from build123d import *

# Parameters (mm, degrees)
SKIZZE1_W                          = 20
SKIZZE1_H                          = 20
AUFSATZ_LINEAR_AUSTRAGEN1_DEPTH    = 15
SKIZZE2_R                          = 2.5
SCHNITT_LINEAR_AUSTRAGEN1_DEPTH    = 7
SKIZZE4_R                          = 4
SCHNITT_LINEAR_AUSTRAGEN7_DEPTH    = 33.015621187
M3X0_5_GEWINDEBOHRUNG1_D           = 2.5
M3X0_5_GEWINDEBOHRUNG1_CSINK_D     = 3.05
M3X0_5_GEWINDEBOHRUNG1_CSINK_ANGLE = 90


with BuildPart() as part:
    # Skizze1 → Aufsatz-Linear austragen1 (new body)
    with BuildSketch(Plane(origin=(0, 0, 0), x_dir=(1, 0, 0), z_dir=(0, 1, 0))):
        with Locations((10, 10)):
            Rectangle(SKIZZE1_W, SKIZZE1_H)
    extrude(amount=AUFSATZ_LINEAR_AUSTRAGEN1_DEPTH)

    # Skizze2 → Schnitt-Linear austragen1 (cut)
    with BuildSketch(Plane.XY):
        with Locations((10, 7.5)):
            Circle(SKIZZE2_R)
    extrude(amount=-SCHNITT_LINEAR_AUSTRAGEN1_DEPTH, mode=Mode.SUBTRACT)

    # Skizze4 → Schnitt-Linear austragen7 (cut, through all)
    with BuildSketch(Plane(origin=(20, 0, 0), x_dir=(0, 0, -1), z_dir=(1, 0, 0))):
        with Locations((13, 7.5)):
            Circle(SKIZZE4_R)
    extrude(amount=-SCHNITT_LINEAR_AUSTRAGEN7_DEPTH, mode=Mode.SUBTRACT)

    # M3x0.5 Gewindebohrung1 (through all)
    with Locations(Plane(origin=(12, 15, 0), x_dir=(0, 0, 1), z_dir=(0, 1, 0))):
        with Locations((-3.5, -2), (-13, -2)):
            CounterSinkHole(M3X0_5_GEWINDEBOHRUNG1_D / 2, M3X0_5_GEWINDEBOHRUNG1_CSINK_D / 2, counter_sink_angle=M3X0_5_GEWINDEBOHRUNG1_CSINK_ANGLE)


solid = part.part
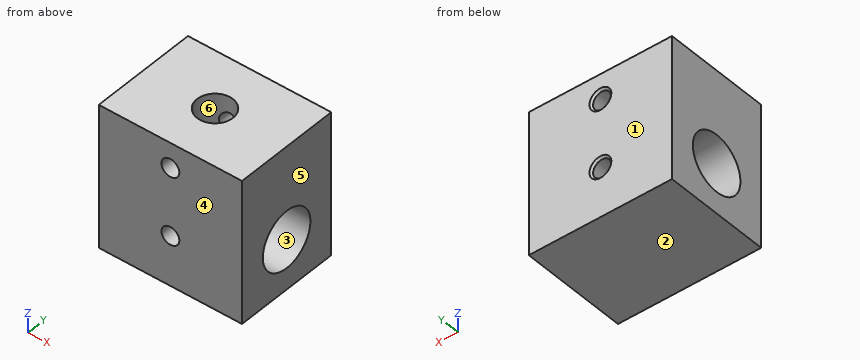
Part model, mm, in its own coordinate system. Face numbers are marked on the shaded views. A direction names the side the tool comes from. Give positions to 0.01 mm unless a question says otherwise; leave off trailing zeros. Loops run counter-clockwise (first coordinate to the right, second up) from the corner with the lowest first, then second, coordinate; pieces in that order, holes last.
(1) Band-saw the part on B-B (x = 10). Write the cut outline in (y, z) (3 decimals).
Return value:
outline: (0, -20) - (15, -20) - (15, -14.525) - (14.725, -14.25) - (11.3, -14.25) arc R4 cw to (3.7, -14.25) - (0, -14.25) - close; (0, -11.75) - (3.7, -11.75) arc R4 cw to (11.3, -11.75) - (14.725, -11.75) - (15, -11.475) - (15, -5.025) - (14.725, -4.75) - (10, -4.75) - (10, -7) - (5, -7) - (5, -4.75) - (0, -4.75) - close; (0, -2.25) - (5, -2.25) - (5, 0) - (0, 0) - close; (10, -2.25) - (14.725, -2.25) - (15, -1.975) - (15, 0) - (10, 0) - close
(2) Band-saw the part on A-A (y = 7.5). Write the cut outline in (x, z).
Return value:
outline: (0, -20) - (20, -20) - (20, -17) - (0, -17) - close; (0, -9) - (20, -9) - (20, 0) - (12.5, 0) - (12.5, -7) - (7.5, -7) - (7.5, 0) - (0, 0) - close
(3) Pull direction Y, two halves, no side cores. Call the marked faces 1, 2, 3 and 4: pulls with the +Y half, pulls with the -Y half, needs draft (parallel to the pull), parting line crosses it, or undercut.
Return value:
face 1: pulls with the +Y half
face 2: needs draft
face 3: undercut
face 4: pulls with the -Y half
(4) Drill centre lines: line 1 along Y through (x, z) = (7, -13); line 2 along X through (y, z) = (12.05, -13); line 3 along Z through (x, y) = (13.75, 6.25). Where is each one in solid material? Low to high.
Return value:
line 1: y = 0 to 3.5, 11.5 to 15
line 2: x = 0 to 8.75, 11.25 to 20
line 3: z = -20 to -16.8, -9.2 to 0
(5) 3-axis set-ups, long thin cutter, end or side, ignore diameter. For the marked faces 5 and 6: which of +Z, -Z, +X, -X, +Y, -Y reach the whole face in a straight line?
Return value:
face 5: +Z, -Z, +X, +Y, -Y
face 6: +Z
(6) Band-saw the part on D-D (x = 6.25). Write the cut outline in (y, z).
Return value:
outline: (0, -20) - (15, -20) - (15, 0) - (0, 0) - close; hole circle Ø8 at (7.5, -13)
(7) Band-saw the part on C-C (z = -3.5). Write the cut outline in (x, y) (3 decimals), and give its area (3 significant figures).
Return value:
outline: (0, 0) - (8.75, 0) - (8.75, 5.335) arc R2.5 cw to (8.75, 9.665) - (8.75, 14.725) - (8.475, 15) - (0, 15) - close; (11.25, 0) - (20, 0) - (20, 15) - (11.525, 15) - (11.25, 14.725) - (11.25, 9.665) arc R2.5 cw to (11.25, 5.335) - close
area: 255 mm2
(8) Pin check, flat tips, straight feed: pin 1 (7 mm diameter, centred on y = 7.5, z = -13, fed in from -X); pin 2 (2.5 mm diameter, centred on x = 9.5, y = 7.5, fed in from +Z). Stop position of each tip, or through.
Return value:
pin 1: passes through
pin 2: stops at z = -7
